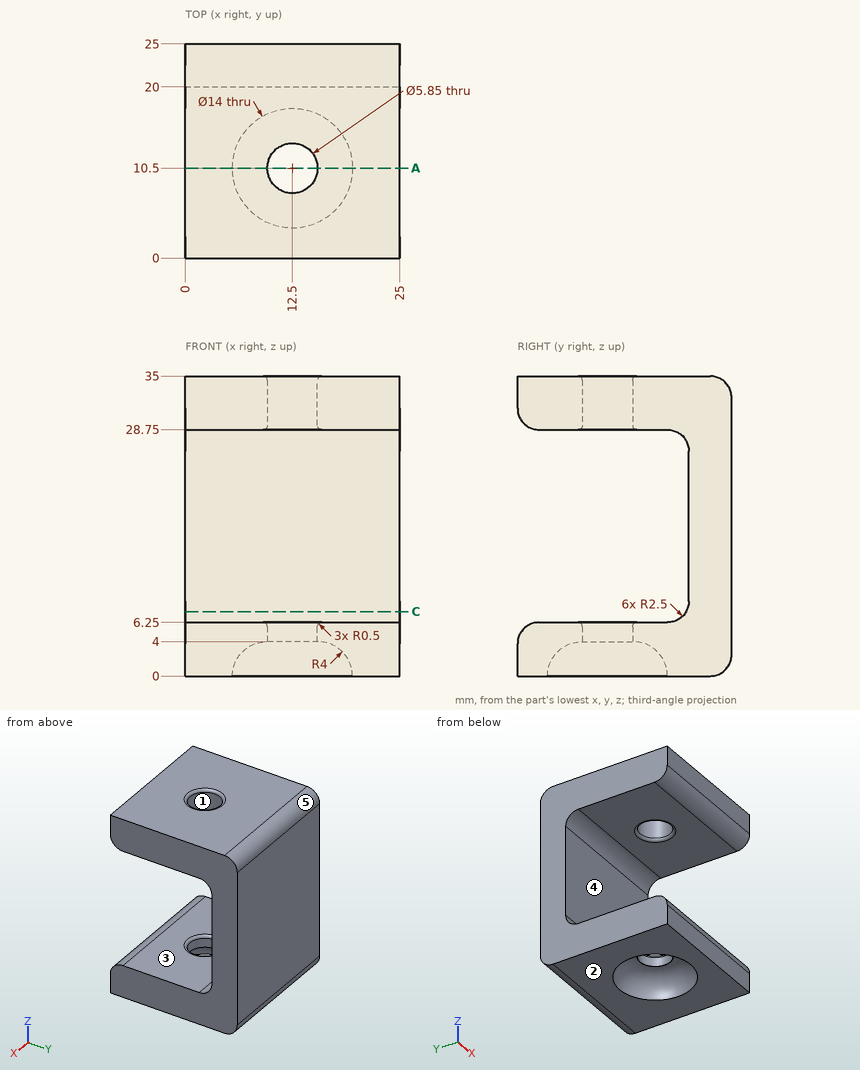
Geometry check sheet. Reference: drawing and pictorial views, mm from the part's lowest x, y, z. A direction names the side the tool comes from. Round coordinates to 2 decimals unless told otherwise and drop trailing zeros. Loops run counter-clockwise (first coordinate to the right, second up) from the corner with the lowest first, then second, coordinate; pieces in that order, holes last. Notation, with made-up numbers: (83, 8) -> (140, 8) arc R33 ccw to (140, 42) -> close; hole circle Ø10 at (35.25, -20). An arc over 180 degrees is marked (long way). Answer as a JSON object with one key per item and string values.
Q1. Section check C-C (z = 7.5). Record the boundary of the cut face in (x, y), then the cut area to 3 significant figures.
Data:
{"outline": "(0, 19.67) -> (25, 19.67) -> (25, 25) -> (0, 25) -> close", "area": "133 mm2"}
Q2. Access from +Z, -Z, +X, -X, +Y, -Y to the whole of each face (thin tool, end or side, straight path). Record for the marked faces 4 and 5.
Data:
{"face 4": "+X, -X, -Y", "face 5": "+Z, +X, -X, +Y"}
Q3. Go/stop test with flat-tipped pins: P1, Ø12, axis at y = 15.5, z = 27, coming from the +X side; P2, Ø6.5, axis at x = 12.5, y = 10.5, coming from the +Z side; P3, Ø7.5, axis at x = 12.5, y = 10.5, coming from the -Z side; P4, Ø7.5, axis at x = 13.5, y = 12.5, coming from the -Z side. Record where each tip stops, or that it passes through.
Data:
{"P1": "stops at x = 25", "P2": "stops at z = 34.97", "P3": "stops at z = 3.93", "P4": "stops at z = 2.66"}
Q4. Scan lines: line 1 (X direction, y = 10.5, z = 4.7) (3 decimals); line 2 (Z direction, x = 22, y = 14.75); line 3 (Z direction, x = 16.25, y = 12.75). Record each from-to range of solid material in increasing order. Write a range as from..to.
Data:
{"line 1": "x = 0..9.575, 15.425..25", "line 2": "z = 0..6.25, 28.75..35", "line 3": "z = 3.76..6.25, 28.75..35"}
Q5. Section check A-A (y = 10.5). State how many separate pieces and enclosed holes the cut face has, then the cut area to 3 significant figures.
Data:
{"separate pieces": "4", "enclosed holes": "0", "area": "213 mm2"}
Q6. Draft check along Z on the marked faces 1, 2 and 3. Enter one of: pulls with the +Z half, pulls with the -Z half, needs draft (parallel to the pull), parting line crosses it, or undercut.
Data:
{"face 1": "needs draft", "face 2": "pulls with the -Z half", "face 3": "undercut"}
